Can you work these out from the model? Positions are in its coordinate system, mm. A direction names the side the tool comes from. Round coordinates to 2 decimals unless told otherwise and drop trailing zeros. Loops run counter-clockwise (first coordinate to the right, second up) from the corner with the lowest first, then second, coordinate; pieces in that order, holes last.
(1) If I drill on line 1 along X through (y, z) = (0.95, 0); line 2 along Y through (x, z) = (-21.5, 5); line 3 along Z through (x, y) = (2, 5.75), over which ranges is the centre line in solid material (lowest first)?
(2) I want a section at C-C on y = 2.25. Write out the boundary of the cut face in (x, z), plus the area to 3 significant figures.
(3) Will these pins go through, and if not, where does the flat tip stop? pin 1 Ø12 at (x, z) = (10.5, -8) entering from -Y; pin 2 Ø4 at (y, z) = (3, -5.5) entering from -X; pin 3 Ø5 at (x, y) = (3.5, 4) entering from -Z; pin 4 Ø21 at (x, z) = (13, -4.5) entering from -Y.
(4) I want a section at A-A on x = -4. Write out the boundary of the cut face in (y, z).
(5) I want a section at B-B on z = 0. Write out the boundary of the cut face in (x, y), plus the area to 3 significant figures.
(6) Thinking about a two-plate mould opening in Z: for faces 4 (the face through (-22.4, -3, 0.1)), 5 (the face through (2, -2, -24)), which applies, released by +Z, released by -Z, zero draft, split by the parting line, or undercut?
(7) Which directions (+Z, -Z, +X, -X, +Y, -Y) give clear straight access to the entire face, cutting with the end or side of a thin tool? Please do faces 1 (the face through (2, -2, 24)), 2 (the face through (-23, 8.5, -6)), 3 (the face through (15.88, 4.95, -17.32)).
from build123d import *

# Parameters (mm, degrees)
SKETCH1_R           = 23.5
SKETCH1_R_2         = 22
BOSS_EXTRUDE1_DEPTH = 1.5
SKETCH2_R           = 26
SKETCH2_R_2         = 23.5
BOSS_EXTRUDE2_DEPTH = 8.5
BOSS_EXTRUDE3_START = 3
BOSS_EXTRUDE3_DEPTH = 3


with BuildPart() as part:
    # Sketch1 → Boss-Extrude1 (new body)
    with BuildSketch(Plane(origin=(0, 0, 0), x_dir=(1, 0, 0), z_dir=(0, 1, 0))):
        with Locations(Location((0, 0, 0), (0, 0, 270))):
            Circle(SKETCH1_R)
        with Locations(Location((0, 0, 0), (0, 0, 270))):
            Circle(SKETCH1_R_2, mode=Mode.SUBTRACT)
    extrude(amount=BOSS_EXTRUDE1_DEPTH)

    # Sketch2 → Boss-Extrude2 (add)
    with BuildSketch(Plane(origin=(0, 0, 0), x_dir=(1, 0, 0), z_dir=(0, 1, 0))):
        with Locations(Location((0, 0, 0), (0, 0, 270))):
            Circle(SKETCH2_R)
        with Locations(Location((0, 0, 0), (0, 0, 270))):
            Circle(SKETCH2_R_2, mode=Mode.SUBTRACT)
    extrude(amount=BOSS_EXTRUDE2_DEPTH)

    # Sketch3 → Boss-Extrude3 (add)
    with BuildSketch(Plane.XZ.offset(BOSS_EXTRUDE3_START)):
        with BuildLine():
            ThreePointArc((0, 26), (-26, 0), (0, -26))
            ThreePointArc((0, -26), (2, -24), (0, -22))
            ThreePointArc((0, -22), (-22, 0), (0, 22))
            ThreePointArc((0, 22), (2, 24), (0, 26))
        make_face()
    extrude(amount=-BOSS_EXTRUDE3_DEPTH)


solid = part.part
Filled sheet:
1. line 1: x = -26 to -22, 22 to 26
1. line 2: y = -3 to 1.5
1. line 3: z = -25.92 to -23.41, 23.41 to 25.92
2. outline: circle Ø52 at (0, 0); hole circle Ø47 at (0, 0)
2. area: 389 mm2
3. pin 1: passes through
3. pin 2: stops at x = -25.76
3. pin 3: stops at z = -25.98
3. pin 4: stops at y = 0
4. outline: (-3, -25.69) - (8.5, -25.69) - (8.5, -23.16) - (1.5, -23.16) - (1.5, -21.63) - (-3, -21.63) - close; (-3, 21.63) - (1.5, 21.63) - (1.5, 23.16) - (8.5, 23.16) - (8.5, 25.69) - (-3, 25.69) - close
5. outline: (-26, -3) - (-22, -3) - (-22, 1.5) - (-23.5, 1.5) - (-23.5, 8.5) - (-26, 8.5) - close; (22, 0) - (26, 0) - (26, 8.5) - (23.5, 8.5) - (23.5, 1.5) - (22, 1.5) - close
5. area: 59.0 mm2
6. face 4: zero draft
6. face 5: undercut
7. face 1: +X, -Y
7. face 2: +Z, -Z, +X, -X, +Y
7. face 3: +Y
